```python
from build123d import *

# Parameters (mm, degrees)
F1_DEPTH = 6.3754
F2_DEPTH = 2.54


with BuildPart() as f1:
    # F0 (on Front) → F1 (new body)
    with BuildSketch(Plane.XZ):
        Polygon((35.56, 54.4186271727), (22.86, 23.7581149306), (27.94, 11.4939100337), (45.72, 54.4186271727), align=None)
        Polygon((22.86, 23.7581149306), (10.16, 54.4186271727), (0, 54.4186271727), (17.78, 11.4939100337), align=None)
        Polygon((27.94, 11.4939100337), (22.86, 23.7581149306), (17.78, 11.4939100337), (22.86, -0.7702948631), align=None)
        Polygon((45.7218143962, -31.4351874453), (27.94, 11.4939100337), (22.86, -0.7702948631), (35.56, -31.4308071053), align=None)
        Polygon((22.86, -0.7702948631), (17.78, 11.4939100337), (0, -31.4308071053), (10.16, -31.4308071053), align=None)
    extrude(amount=F1_DEPTH)

    # F2 (cut): a face of the model
    f2_faces = [f1.faces().sort_by_distance(p)[0] for p in [
        (22.8602675118, -6.3754, 11.4933203606),
    ]]
    extrude(f2_faces, amount=-F2_DEPTH, mode=Mode.SUBTRACT)


solid = f1.part
```
Model file for the job. Use its own axes, mm. A direction names the side the tool comes from. Give positions to 0.01 mm unless a question says otherwise; leave off trailing zeros. Order: outer loops, then holes, each group sorted by start corner. A loop starts at its lowest first (then second) coordinate and runs counter-clockwise, first axis right, second up.
1) Wall check: probe 1 along Z at (x, y) = (30.5, -0.65); probe 2 along Z at (x, y) = (16, -2.55); probe 3 along X at (y, z) = (-0.95, -15). Give the ranges that are in metal, low to high.
2) Saw through at A-A, the plane z = 48. Write the cut outline in (x, y).
3) Pin check, flat tips, straight feed: pin 1 (1.9 mm diameter, centred on x = 7.5, y = -1, fed in from -Z); pin 2 (1.5 mm diameter, centred on x = 15, y = -1.5, fed in from +Z); pin 3 (8 mm diameter, centred on x = 14, z = -20, fed in from +Y). Stop position of each tip, or through.
4) Saw through at B-B, the plane x = 4. Write the cut outline in (y, z), then the cut area to 3 significant figures.
5) Saw through at C-C, the plane y = -1. Write the cut outline in (x, z).
6) 3-axis set-ups, long thin cutter, end or side, ignore diameter. For faces 1 (the flat face through (29.299, -1.891, 39.303)), 2 (the flat face through (9, -1.9, -9.7)), 3 (the flat face through (36.706, -1.891, 32.656)), 4 (the flat face through (29.121, -1.891, -15.886)): which of +Z, -Z, +X, -X, +Y, -Y reach the whole face in a straight line?
7) Saw through at D-D, the plane x = 22. Write the cut outline in (y, z), then the cut area to 3 significant figures.
Computed:
1. probe 1: z = -19.21 to 5.31, 17.67 to 42.2
1. probe 2: z = -17.33 to 7.2, 15.79 to 40.32
1. probe 3: x = 6.81 to 16.97, 28.75 to 38.91
2. outline: (2.66, -3.84) - (12.82, -3.84) - (12.82, 0) - (2.66, 0) - close; (32.9, -3.84) - (43.06, -3.84) - (43.06, 0) - (32.9, 0) - close
3. pin 1: stops at z = -31.43
3. pin 2: stops at z = 44.54
3. pin 3: stops at y = 0
4. outline: (-3.84, -31.43) - (0, -31.43) - (0, -21.77) - (-3.84, -21.77) - close; (-3.84, 44.76) - (0, 44.76) - (0, 54.42) - (-3.84, 54.42) - close
4. area: 74.1 mm2
5. outline: (0, -31.43) - (10.16, -31.43) - (22.86, -0.77) - (35.56, -31.43) - (45.72, -31.44) - (27.94, 11.49) - (45.72, 54.42) - (35.56, 54.42) - (22.86, 23.76) - (10.16, 54.42) - (0, 54.42) - (17.78, 11.49) - close
6. face 1: +Z, +Y, -Y
6. face 2: -X, +Y, -Y
6. face 3: +X, +Y, -Y
6. face 4: -Z, +Y, -Y
7. outline: (-3.84, -2.85) - (0, -2.85) - (0, 25.83) - (-3.84, 25.83) - close
7. area: 110 mm2
